from build123d import *

# Parameters (mm, degrees)
SKETCH1_R           = 14.6
BOSS_EXTRUDE1_DEPTH = 3
SHELL2_T            = 1
SKETCH2_W           = 2.2
SKETCH2_H           = 4.2
BOSS_EXTRUDE2_DEPTH = 5
SHELL3_T            = 1.2
SKETCH3_R           = 8
CUT_EXTRUDE1_DEPTH  = 25.06075643


with BuildPart() as part:
    # Sketch1 → Boss-Extrude1 (new body)
    with BuildSketch(Plane(origin=(0, 0, 0), x_dir=(1, 0, 0), z_dir=(0, 1, 0))):
        with Locations(Location((0, 0, 0), (0, 0, 270))):
            Circle(SKETCH1_R)
    extrude(amount=BOSS_EXTRUDE1_DEPTH)

    # Shell2
    shell2_openings = [part.faces().sort_by_distance(p)[0] for p in [
        (0, 3, 0),
    ]]
    offset(amount=SHELL2_T, openings=shell2_openings, kind=Kind.INTERSECTION)

    # Sketch2 → Boss-Extrude2 (add)
    with BuildSketch(Plane(origin=(0, 0, 0), x_dir=(1, 0, 0), z_dir=(0, 1, 0))):
        with Locations((8.6, 0)):
            Rectangle(SKETCH2_W, SKETCH2_H)
    extrude(amount=BOSS_EXTRUDE2_DEPTH)

    # Shell3
    shell3_openings = [part.faces().sort_by_distance(p)[0] for p in [
        (8.6, 5, 0),
    ]]
    offset(amount=SHELL3_T, openings=shell3_openings, kind=Kind.INTERSECTION)

    # Sketch3 → Cut-Extrude1 (cut, through all)
    with BuildSketch(Plane(origin=(0, 1.2, 0), x_dir=(1, 0, 0), z_dir=(0, 1, 0))):
        with Locations(Location((-3, 0, 0), (0, 0, 270))):
            Circle(SKETCH3_R)
    extrude(amount=-CUT_EXTRUDE1_DEPTH, mode=Mode.SUBTRACT)


solid = part.part
Verification items for the finished model (mm, model axes). A direction names the side the tool comes from. Give positions to 0.01 mm unless a question says otherwise; leave off trailing zeros. Write each loop counter-clockwise with the first axis right and the second up, starting at its lowest first coordinate (ties: lowest second). Pieces come first, ordered by that corner, then holes. Notation, with made-up numbers: (29, -27) - (79, -27) arc R29 cw to (79, 10) - close; hole circle Ø10 at (52.25, -8). An arc over 180 degrees is marked (long way). Answer as CSV lines item,"result". Start each with the question number.
1. Sectioned sample at A-A (z = 0). Count the separate pieces of the cut face and the enclosed holes in it, then the cut area to 3 significant figures.
2. Sectioned sample at C-C (z = 14). Record the boundary of the cut face in (x, y), then the cut area to 3 significant figures.
3. Draft check along Z on faces 4 (the face through (9, 2, 2.1)), 5 (the face through (2.4, -1.6, -5.9)), 6 (the face through (5.046, 0.955, 16.024)), 7 (the face through (-5, 4.2, -13)). Enter one of: pulls with the +Z half, pulls with the -Z half, needs draft (parallel to the pull), parting line crosses it, or undercut.
4. Set-up check for faces 1 (the face through (9, 3, -3.3)), 2 (the face through (-14, 3, 6)), 3 (the face through (8, -2.2, 0)): record each of +Z, -Z, +X, -X, +Y, -Y from which the full face is reachable in a straight line by a thin tool's end or side.
5. Sectioned sample at D-D (x = 1). Record the boundary of the cut face in (y, z).
6. Thickness scan on line 1 (X direction, y = 0.8, z = 0); line 2 (Y direction, x = -14.5, z = 4.5); line 3 (X direction, y = -1.6, z = 0). Record the ranges inside material, lowest first.
7. Sectioned sample at B-B (x = 7). Record the boundary of the cut face in (y, z).
8. Depth check by flat-ended pin: pin 1 (4 mm diameter, centred on y = 2.5, z = -6.5, fed in from +X); pin 2 (2.5 mm diameter, centred on x = 8.5, y = 1.5, fed in from +Z); pin 3 (6 mm diameter, centred on x = -2.5, z = -12, fed in from +Y); pin 4 (14.5 mm diameter, centred on x = -3, z = 0, fed in from -Y). Enter the tip coordinate at first touch or a pass-through.
Derived:
1,separate pieces,"3"
1,enclosed holes,"0"
1,area,"65.5 mm²"
2,outline,"(-9.29, -2.2) - (9.29, -2.2) - (9.29, 4.2) - (-9.29, 4.2) - close; hole (-6.88, -1) - (6.88, -1) - (6.88, 3) - (4.14, 3) - (4.14, 0) - (-4.14, 0) - (-4.14, 3) - (-6.88, 3) - close"
2,area,"88.7 mm²"
3,face 4,"undercut"
3,face 5,"undercut"
3,face 6,"parting line crosses it"
3,face 7,"needs draft"
4,face 1,"+Y"
4,face 2,"none"
4,face 3,"+Z, -Z, +X, -X, -Y"
5,outline,"(-2.2, -16.77) - (4.2, -16.77) - (4.2, -13.36) - (1.2, -13.36) - (1.2, -6.93) - (0, -6.93) - (0, -14.57) - (3, -14.57) - (3, -15.57) - (-1, -15.57) - (-1, -6.93) - (-2.2, -6.93) - close; (-2.2, 6.93) - (-1, 6.93) - (-1, 15.57) - (3, 15.57) - (3, 14.57) - (0, 14.57) - (0, 6.93) - (1.2, 6.93) - (1.2, 13.36) - (4.2, 13.36) - (4.2, 16.77) - (-2.2, 16.77) - close"
6,line 1,"-16.8 to -15.6, -14.6 to -11, 5 to 7.5, 9.7 to 14.6, 15.6 to 16.8"
6,line 2,"-2.2 to -1, 3 to 4.2"
6,line 3,"-16.8 to -11, 5 to 16.8"
7,outline,"(-2.2, -15.27) - (4.2, -15.27) - (4.2, -11.43) - (1.2, -11.43) - (1.2, -3.3) - (5, -3.3) - (5, 3.3) - (1.2, 3.3) - (1.2, 11.43) - (4.2, 11.43) - (4.2, 15.27) - (-2.2, 15.27) - close; hole (-1, -13.94) - (3, -13.94) - (3, -12.81) - (0, -12.81) - (0, 12.81) - (3, 12.81) - (3, 13.94) - (-1, 13.94) - close"
8,pin 1,"x = 16.19"
8,pin 2,"z = 15.16"
8,pin 3,"y = 4.2"
8,pin 4,"through"
